from build123d import *

# Parameters (mm, degrees)
EXTRUDE_1_DEPTH = 5


with BuildPart() as part:
    # 草图1 → 凸台-拉伸1 (new body)
    with BuildSketch(Plane.XY):
        with BuildLine():
            Line((33.5, -27.5), (-33.5, -27.5))
            ThreePointArc((-33.5, -27.5), (-35.621320344, -26.621320344), (-36.5, -24.5))
            Line((-36.5, -24.5), (-36.5, 24.5))
            ThreePointArc((-36.5, 24.5), (-35.621320344, 26.621320344), (-33.5, 27.5))
            Line((-33.5, 27.5), (33.5, 27.5))
            ThreePointArc((33.5, 27.5), (35.621320344, 26.621320344), (36.5, 24.5))
            Line((36.5, 24.5), (36.5, -24.5))
            ThreePointArc((36.5, -24.5), (35.621320344, -26.621320344), (33.5, -27.5))
        make_face()
        Polygon((-31.5, 2.5), (-31.5, -2.5), (31.5, -2.5), (31.5, 2.5), (2.5, 2.5), (2.5, 17.5), (-2.5, 17.5), (-2.5, 2.5), align=None, mode=Mode.SUBTRACT)
        with BuildLine():
            Line((13.25, 21), (13.25, 12.5))
            ThreePointArc((13.25, 12.5), (16.5, 9.25), (19.75, 12.5))
            Line((19.75, 12.5), (19.75, 21))
            ThreePointArc((19.75, 21), (16.5, 24.25), (13.25, 21))
        make_face(mode=Mode.SUBTRACT)
        with BuildLine():
            Line((-13.25, 21), (-13.25, 12.5))
            ThreePointArc((-13.25, 12.5), (-16.5, 9.25), (-19.75, 12.5))
            Line((-19.75, 12.5), (-19.75, 21))
            ThreePointArc((-19.75, 21), (-16.5, 24.25), (-13.25, 21))
        make_face(mode=Mode.SUBTRACT)
    extrude(amount=EXTRUDE_1_DEPTH)


solid = part.part
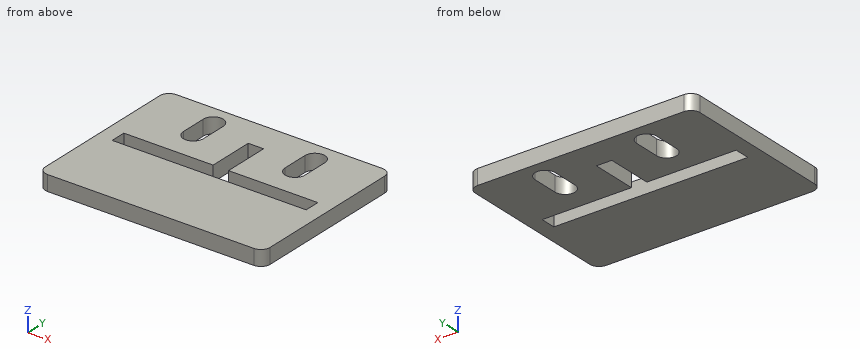
For this review, take the finished solid that the model builds, in its own axes (mm). Give positions to 0.01 mm unless a question says otherwise; leave off trailing zeros. Loops run counter-clockwise (first coordinate to the right, second up) from the corner with the lowest first, then second, coordinate; pieces in that order, holes last. Notation, with made-up numbers: M 24.5,72.5 L 28.5,72.5 A20 ccw 28.5,85.5 Z; hole C 66,86.25 d10. An arc over 180 degrees is marked long. Answer as a JSON object with one key per item and string values. Group by question number.
Q1. Add section D-D on x = -27. Give the boundary of the cut face in (y, z).
Q2. For probe 1 along X at (y, z) = (18, 3.6); probe 2 along X at (y, z) = (15.5, 2.7); probe 3 along Y at (x, z) = (-5, 1), list the stretches that pass through material, from the lowest coordinate up. Write a range as [from, to].
Q3. Add section A-A on y = 1.5. Give the boundary of the cut face in (x, z), and give its area (3 significant figures).
Q4. Add section C-C on x = 16.5. Give the boundary of the cut face in (y, z), and give its area (3 significant figures).
Q5. Add section B-B on z = 4. Give the boundary of the cut face in (x, y), and give its area (3 significant figures).
Checked values:
{
 "1": {"outline": "M -27.5,0 L -2.5,0 L -2.5,5 L -27.5,5 Z; M 2.5,0 L 27.5,0 L 27.5,5 L 2.5,5 Z"},
 "2": {"probe 1": "[-36.5, -19.75], [-13.25, 13.25], [19.75, 36.5]", "probe 2": "[-36.5, -19.75], [-13.25, -2.5], [2.5, 13.25], [19.75, 36.5]", "probe 3": "[-27.5, -2.5], [2.5, 27.5]"},
 "3": {"outline": "M -36.5,0 L -31.5,0 L -31.5,5 L -36.5,5 Z; M 31.5,0 L 36.5,0 L 36.5,5 L 31.5,5 Z", "area": "50.0 mm²"},
 "4": {"outline": "M -27.5,0 L -2.5,0 L -2.5,5 L -27.5,5 Z; M 2.5,0 L 9.25,0 L 9.25,5 L 2.5,5 Z; M 24.25,0 L 27.5,0 L 27.5,5 L 24.25,5 Z", "area": "175 mm²"},
 "5": {"outline": "M -36.5,-24.5 A3 ccw -33.5,-27.5 L 33.5,-27.5 A3 ccw 36.5,-24.5 L 36.5,24.5 A3 ccw 33.5,27.5 L -33.5,27.5 A3 ccw -36.5,24.5 Z; hole M -31.5,-2.5 L 31.5,-2.5 L 31.5,2.5 L 2.5,2.5 L 2.5,17.5 L -2.5,17.5 L -2.5,2.5 L -31.5,2.5 Z; hole M -19.75,12.5 A3.25 ccw -13.25,12.5 L -13.25,21 A3.25 ccw -19.75,21 Z; hole M 13.25,12.5 A3.25 ccw 19.75,12.5 L 19.75,21 A3.25 ccw 13.25,21 Z", "area": "3,440 mm²"}
}
